Can you work these out from the model? Positions are in its coordinate system, mm. A direction names the side the tool comes from. Round coordinates to 2 decimals unless told otherwise and drop trailing zeros. Order: outer loops, then holes, each group sorted by start corner. A loop starts at its lowest first (then second) coordinate and runs counter-clockwise, first axis right, second up.
Q1. If we section it at A-A (x = -15.5): Please give me the cut outline in (y, z), plus the area to 3 significant figures.
Q2. If we section it at C-C (z = 53): Please give me the cut outline in (x, y), plus the area to 3 significant figures.
Q3. If I drill on line 1 (Z direction, x = -33.5, y = 63.5); line 2 (Y direction, x = -28, z = 119.5), over which ranges is the centre line in solid material (lowest first)?
Q4. Will this pin go through, and if not, where does the flat tip stop? P1, Ø1, axis at x = -16, y = 16, coming from the +Z side.
Q5. If we section it at B-B (y = 53): Please give me the cut outline in (x, z), plus the area to 3 significant figures.
Q6. For faces 1 (the face through (-1, -137.16, 68)), 2 (the face through (-1, -21.209, 99)), which set-ups out of +Z, -Z, +X, -X, +Y, -Y let a thin tool reach every point of the face, with its end or its side?
from build123d import *

# Parameters (mm, degrees)
F0_W     = 75.9968
F0_H     = 29.5656
F1_DEPTH = 137.16
F2_W     = 75.9968
F2_H     = 115.951
F3_DEPTH = 138.43
F4_W     = 75.9968
F4_H     = 158.369
F5_DEPTH = 31.496


with BuildPart() as f1:
    # F0 (on Front) → F1 (new body, symmetric)
    with BuildSketch(Plane.XZ):
        Rectangle(F0_W, F0_H)
    extrude(amount=F1_DEPTH, both=True)

    # F2 (on face) → F3 (join)
    with BuildSketch(Plane.XY.offset(14.7828)):
        with Locations((0, -79.1845)):
            Rectangle(F2_W, F2_H)
    extrude(amount=F3_DEPTH)

    # F4 (on face) → F5 (join)
    with BuildSketch(Plane.XY.offset(14.7828)):
        with Locations((0, 57.9755)):
            Rectangle(F4_W, F4_H)
    extrude(amount=F5_DEPTH)


solid = f1.part
Solution:
1. outline: (-137.16, -14.78) - (137.16, -14.78) - (137.16, 46.28) - (-21.21, 46.28) - (-21.21, 153.21) - (-137.16, 153.21) - close
1. area: 29,100 mm2
2. outline: (-38, -137.16) - (38, -137.16) - (38, -21.21) - (-38, -21.21) - close
2. area: 8,810 mm2
3. line 1: z = -14.78 to 46.28
3. line 2: y = -137.16 to -21.21
4. P1: stops at z = 46.28
5. outline: (-38, -14.78) - (38, -14.78) - (38, 46.28) - (-38, 46.28) - close
5. area: 4,640 mm2
6. face 1: +Z, -Z, +X, -X, -Y
6. face 2: +Z, +X, -X, +Y
